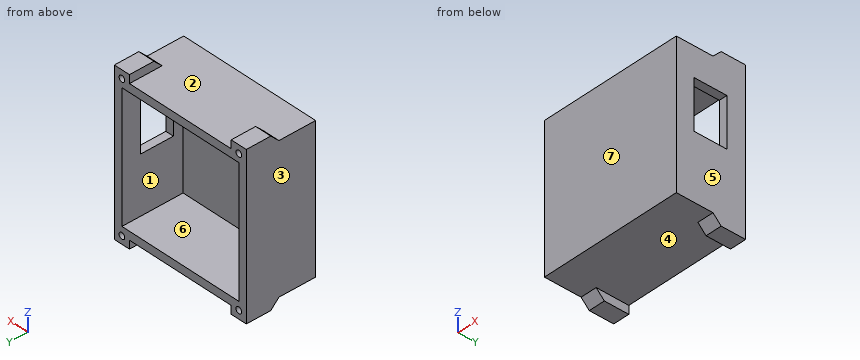
```python
from build123d import *

# Parameters (mm, degrees)
SKETCH1_W           = 35
SKETCH1_H           = 35
SKETCH1_W_2         = 31
SKETCH1_H_2         = 31
BOSS_EXTRUDE1_DEPTH = 2
SKETCH1_3_W         = 35
SKETCH1_3_H         = 35
SKETCH1_3_W_2       = 31
SKETCH1_3_H_2       = 31
BOSS_EXTRUDE2_DEPTH = 17
SKETCH2_W           = 12
SKETCH2_H           = 8
CUT_EXTRUDE1_DEPTH  = 15
SKETCH3_W           = 4
SKETCH3_H           = 2
BOSS_EXTRUDE3_DEPTH = 6
CHAMFER1_SIZE       = 2
SKETCH4_R           = 0.75
CUT_EXTRUDE2_DEPTH  = 6


with BuildPart() as part:
    # Sketch1 → Boss-Extrude1 (new body)
    # profile 1 of 2: a face of its own
    with BuildSketch(Plane(origin=(0, 0, 0), x_dir=(1, 0, 0), z_dir=(0, 1, 0))):
        with Locations((15.5, 15.5)):
            Rectangle(SKETCH1_W, SKETCH1_H)
        with Locations((15.5, 15.5)):
            Rectangle(SKETCH1_W_2, SKETCH1_H_2, mode=Mode.SUBTRACT)
    # profile 2 of 2: a face of its own
    with BuildSketch(Plane(origin=(0, 0, 0), x_dir=(1, 0, 0), z_dir=(0, 1, 0))):
        with Locations((15.5, 15.5)):
            Rectangle(SKETCH1_W_2, SKETCH1_H_2)
    extrude(amount=BOSS_EXTRUDE1_DEPTH)

    # Sketch1<3> → Boss-Extrude2 (add)
    with BuildSketch(Plane(origin=(0, 0, 0), x_dir=(1, 0, 0), z_dir=(0, 1, 0))):
        with Locations((15.5, 15.5)):
            Rectangle(SKETCH1_3_W, SKETCH1_3_H)
        with Locations((15.5, 15.5)):
            Rectangle(SKETCH1_3_W_2, SKETCH1_3_H_2, mode=Mode.SUBTRACT)
    extrude(amount=BOSS_EXTRUDE2_DEPTH)

    # Sketch2 → Cut-Extrude1 (cut)
    with BuildSketch(Plane(origin=(33, 0, 0), x_dir=(0, 0, -1), z_dir=(1, 0, 0))):
        with Locations((11.111303283, 8.4)):
            Rectangle(SKETCH2_W, SKETCH2_H)
    extrude(amount=-CUT_EXTRUDE1_DEPTH, mode=Mode.SUBTRACT)

    # Sketch3 → Boss-Extrude3 (add)
    with BuildSketch(Plane(origin=(0, 17, 0), x_dir=(1, 0, 0), z_dir=(0, 1, 0))):
        with Locations((31, 34)):
            Rectangle(SKETCH3_W, SKETCH3_H)
        with Locations((0, 34)):
            Rectangle(SKETCH3_W, SKETCH3_H)
        with Locations((0, -3)):
            Rectangle(SKETCH3_W, SKETCH3_H)
        with Locations((31, -3)):
            Rectangle(SKETCH3_W, SKETCH3_H)
    extrude(amount=-BOSS_EXTRUDE3_DEPTH)

    # Chamfer1
    chamfer1_edges = [part.edges().sort_by_distance(p)[0] for p in [
        (31, 11, 2),
        (0, 11, 2),
        (0, 11, -33),
        (31, 11, -33),
    ]]
    chamfer(chamfer1_edges, length=CHAMFER1_SIZE - 0.0001)  # a hair under: the kernel refuses the full size

    # Sketch4 → Cut-Extrude2 (cut)
    with BuildSketch(Plane(origin=(0, 17, 0), x_dir=(1, 0, 0), z_dir=(0, 1, 0))):
        with Locations(Location((31, 33.122538924, 0), (0, 0, 270))):
            Circle(SKETCH4_R)
        with Locations(Location((31, -2, 0), (0, 0, 270))):
            Circle(SKETCH4_R)
        with Locations(Location((0, -2, 0), (0, 0, 270))):
            Circle(SKETCH4_R)
        with Locations(Location((0, 33, 0), (0, 0, 270))):
            Circle(SKETCH4_R)
    extrude(amount=-CUT_EXTRUDE2_DEPTH, mode=Mode.SUBTRACT)


solid = part.part
```
Geometry check sheet. Reference: the model listing, model coordinates, mm. Face numbers are marked on the shaded views. A direction names the side the tool comes from. Give positions to 0.01 mm unless a question says otherwise; leave off trailing zeros. Write each loop counter-clockwise with the first axis right and the second up, starting at its lowest first coordinate (ties: lowest second). Pieces come first, ordered by that corner, then holes.
1) Section check B-B, the plane z = -12. Record the boundary of the cut face in (x, y), and give its area (3 significant figures).
2) Section check A-A, the plane y = 3. Record the boundary of the cut face in (x, z), and give its area (3 significant figures).
3) Section check D-D, the plane z = -1. Record the boundary of the cut face in (x, y), and give its area (3 significant figures).
4) Section check C-C, the plane x = 13. Record the boundary of the cut face in (y, z), and give its area (3 significant figures).
5) Gauge pin test, flat ends, axial feed: pin 1 (10 mm diameter, centred on x = 8, y = 14.5, fed in from +Z); pin 2 (4 mm diameter, centred on x = 4.5, y = 7.5, fed in from -Z); pin 3 (15.5 mm diameter, centred on x = 21.5, z = -15, fed in from +Y). Record the tip position at first contact, or that the pin passes through.
6) Access from +Z, -Z, +X, -X, +Y, -Y to the whole of each face (thin tool, end or side, straight path). Record for the marked faces 1, 2 and 3.
7) Material ranges on L1, parallel to X at y = 4.75, z = -1; L2, parallel to Z at x = 8, y = 14.25; L3, parallel to Y at x = 23.5, z = -3, recorded low to high.
8) Release check for a two-part mould opening along X. For the marked faces 4, 5, 6 and 7 record: pulls with the +X half, pulls with the -X half, needs draft (parallel to the pull), parting line crosses it, or undercut.
Computed:
1. outline: (-2, 0) - (33, 0) - (33, 4.4) - (31, 4.4) - (31, 2) - (0, 2) - (0, 17) - (-2, 17) - close; (31, 12.4) - (33, 12.4) - (33, 17) - (31, 17) - close
1. area: 114 mm2
2. outline: (-2, -33) - (33, -33) - (33, 2) - (-2, 2) - close; hole (0, -31) - (31, -31) - (31, 0) - (0, 0) - close
2. area: 264 mm2
3. outline: (-2, 0) - (33, 0) - (33, 17) - (31, 17) - (31, 2) - (0, 2) - (0, 17) - (-2, 17) - close
3. area: 130 mm2
4. outline: (0, -33) - (17, -33) - (17, -31) - (2, -31) - (2, 0) - (17, 0) - (17, 2) - (0, 2) - close
4. area: 130 mm2
5. pin 1: stops at z = 2
5. pin 2: stops at z = -33
5. pin 3: stops at y = 2
6. face 1: +Y
6. face 2: +Z, -Y
6. face 3: +Z, -Z, -X, +Y, -Y
7. L1: x = -2 to 0, 31 to 33
7. L2: z = -33 to -31, 0 to 2
7. L3: y = 0 to 2
8. face 4: undercut
8. face 5: pulls with the +X half
8. face 6: undercut
8. face 7: needs draft
